from build123d import *

# Parameters (mm, degrees)
SKETCH1_R           = 1
BOSS_EXTRUDE1_DEPTH = 3.175


with BuildPart() as part:
    # Sketch1 → Boss-Extrude1 (new body)
    with BuildSketch(Plane(origin=(0, 0, 0), x_dir=(1, 0, 0), z_dir=(0, 1, 0))):
        with BuildLine():
            Line((-268.253734697, -101.056878234), (-268.253734697, -167.076622113))
            ThreePointArc((-268.253734697, -167.076622113), (-264.197163616, -176.870051033), (-254.403734697, -180.926622113))
            Line((-254.403734697, -180.926622113), (-143.66889433, -180.926622113))
            ThreePointArc((-143.66889433, -180.926622113), (-133.87546541, -176.870051033), (-129.81889433, -167.076622113))
            Line((-129.81889433, -167.076622113), (-129.81889433, -107.776622113))
            ThreePointArc((-129.81889433, -107.776622113), (-133.87546541, -97.983193194), (-143.66889433, -93.926622113))
            Line((-143.66889433, -93.926622113), (-221.881483076, -93.926622113))
            ThreePointArc((-221.881483076, -93.926622113), (-225.7083174, -93.165417438), (-228.952550888, -90.997689925))
            Line((-228.952550888, -90.997689925), (-231.967047619, -87.983193194))
            ThreePointArc((-231.967047619, -87.983193194), (-236.460311001, -84.980890588), (-241.760476539, -83.926622113))
            Line((-241.760476539, -83.926622113), (-251.123478576, -83.926622113))
            ThreePointArc((-251.123478576, -83.926622113), (-256.423644114, -84.980890588), (-260.916907495, -87.983193194))
            Line((-260.916907495, -87.983193194), (-264.197163616, -91.263449315))
            ThreePointArc((-264.197163616, -91.263449315), (-267.199466222, -95.756712696), (-268.253734697, -101.056878234))
        make_face()
        with Locations(Location((-246.441977557, -177.176622113, 0), (0, 0, 270))):
            Circle(SKETCH1_R, mode=Mode.SUBTRACT)
        with Locations(Location((-264.503734697, -133.066750174, 0), (0, 0, 270))):
            Circle(SKETCH1_R, mode=Mode.SUBTRACT)
        with Locations(Location((-246.441977557, -87.676622113, 0), (0, 0, 270))):
            Circle(SKETCH1_R, mode=Mode.SUBTRACT)
        with Locations(Location((-191.484546698, -97.676622113, 0), (0, 0, 270))):
            Circle(SKETCH1_R, mode=Mode.SUBTRACT)
        with Locations(Location((-136.52711584, -100.634843623, 0), (0, 0, 270))):
            Circle(SKETCH1_R, mode=Mode.SUBTRACT)
        with Locations(Location((-136.52711584, -174.218400603, 0), (0, 0, 270))):
            Circle(SKETCH1_R, mode=Mode.SUBTRACT)
        with Locations(Location((-191.484546698, -177.176622113, 0), (0, 0, 270))):
            Circle(SKETCH1_R, mode=Mode.SUBTRACT)
    extrude(amount=BOSS_EXTRUDE1_DEPTH)


solid = part.part
Verification items for the finished model (mm, model axes). A direction names the side the tool comes from. Give positions to 0.01 mm unless a question says otherwise; leave off trailing zeros. Write each loop counter-clockwise with the first axis right and the second up, starting at its lowest first coordinate (ties: lowest second). Pieces come first, ordered by that corner, then holes. Notation, with made-up numbers: M -13,52 L 30,52 A7 ccw 30,59 Z; hole C -2,36 d1. An arc over 180 degrees is marked long. Put each result on its own line as item: value. Start each with the question number.
1. Go/stop test with a flat-tipped pin: pin 1 Ø12 at (x, z) = (-232, 139) entering from -Y. Record where the tip stops, or that it passes through.
2. Section check A-A (y = 2.25). Record the cut outline in (x, z), and give its area (3 significant figures).
3. Section check B-B (x = -153.5). Record the cut outline in (y, z) (3 decimals), and give its area (3 significant figures).
4. Scan lines: line 1 along Z through (x, y) = (-246.5, 2.5); line 2 along X through (y, z) = (0.4, 176.5); line 3 along Z through (x, y) = (-145, 0.1). Record each from-to range of solid material in increasing order. Write a range as [from, to].
5. Section check C-C (x = -230.5). Record the cut outline in (y, z) (3 decimals), and give its area (3 significant figures).
6. Set-up check for faces 1 (the face through (-267.17, 1.57, 95.69)), 2 (the face through (-182, 2, 93.927)): record each of +Z, -Z, +X, -X, +Y, -Y from which the full face is reachable in a straight line by a thin tool's end or side.
Answer list:
1. pin 1: y = 0
2. outline: M -268.25,101.06 A13.85 ccw -264.2,91.26 L -260.92,87.98 A13.85 ccw -251.12,83.93 L -241.76,83.93 A13.85 ccw -231.97,87.98 L -228.95,91 A10 cw -221.88,93.93 L -143.67,93.93 A13.85 ccw -129.82,107.78 L -129.82,167.08 A13.85 ccw -143.67,180.93 L -254.4,180.93 A13.85 ccw -268.25,167.08 Z; hole C -264.5,133.07 d2; hole C -246.44,87.68 d2; hole C -246.44,177.18 d2; hole C -191.48,97.68 d2; hole C -191.48,177.18 d2; hole C -136.53,100.63 d2; hole C -136.53,174.22 d2
2. area: 12,200 mm2
3. outline: M 0,93.927 L 3.175,93.927 L 3.175,180.927 L 0,180.927 Z
3. area: 276 mm2
4. line 1: [83.93, 86.68], [88.67, 176.18], [178.17, 180.93]
4. line 2: [-264.55, -247.18], [-245.71, -192.22], [-190.75, -133.52]
4. line 3: [93.93, 180.93]
5. outline: M 0,89.45 L 3.175,89.45 L 3.175,180.927 L 0,180.927 Z
5. area: 290 mm2
6. face 1: -Z, -X, +Y, -Y
6. face 2: -Z, +X, +Y, -Y
